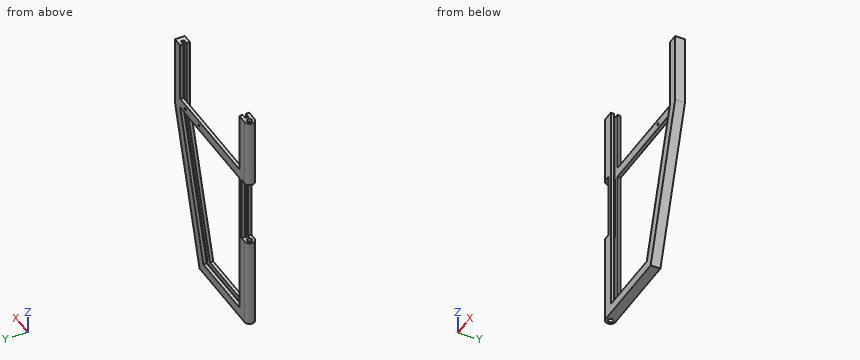
```python
from build123d import *

# Parameters (mm, degrees)
EXTRUDE_1_DEPTH                   = 3
SKETCH_2_R                        = 1.5
SKETCH_2_R_2                      = 0.75
EXTRUDE_2_DEPTH                   = 73
SKETCH_3_W                        = 42
SKETCH_3_H                        = 3.5
SKETCH_3_W_2                      = 3.2
SKETCH_3_H_2                      = 20.2
CUT_EXTRUDE_1_DEPTH               = 83.725086884
CUT_EXTRUDE_2_REACH               = 84.028
CUT_EXTRUDE_2_OFFSET_FROM_SURFACE = 1.5
CUT_EXTRUDE_START                 = -1.5
SKETCH_4_W                        = 44.5
SKETCH_4_H                        = 1
SKETCH_4_3_W                      = 22
SKETCH_4_3_H                      = 1
CUT_EXTRUDE_3_DEPTH               = 37.5
SKETCH_5_W                        = 3
SKETCH_5_H                        = 1
EXTRUDE_3_DEPTH                   = 34.5
SKETCH_6_R                        = 0.35
CUT_EXTRUDE_4_DEPTH               = 80.653562381
SKETCH_7_W                        = 24.036657481
SKETCH_7_H                        = 1
CUT_EXTRUDE_5_DEPTH               = 1.5


with BuildPart() as part:
    # 草图1 → 凸台-拉伸1 (new body)
    with BuildSketch(Plane(origin=(0, 0, 0), x_dir=(1, 0, 0), z_dir=(0, 1, 0))):
        Polygon((0, 0), (0, -73), (38.8, -73), (38.8, -47.5), (24.5, 0), align=None)
    extrude(amount=EXTRUDE_1_DEPTH)

    # 草图2 → 凸台-拉伸2 (add)
    # profile 1 of 2: a face of its own
    with BuildSketch(Plane(origin=(0, 0, 0), x_dir=(-1, 0, 0), z_dir=(0, 0, -1))):
        with BuildLine():
            Line((0, 3), (0, 0))
            Line((0, 0), (1.7, 0))
            ThreePointArc((1.7, 0), (0.2, 1.5), (1.7, 3))
            Line((1.7, 3), (0, 3))
        make_face()
    # profile 2 of 2: a face of its own
    with BuildSketch(Plane(origin=(0, 0, 0), x_dir=(-1, 0, 0), z_dir=(0, 0, -1))):
        with Locations((1.7, 1.5)):
            Circle(SKETCH_2_R)
        with Locations((1.7, 1.5)):
            Circle(SKETCH_2_R_2, mode=Mode.SUBTRACT)
    extrude(amount=-EXTRUDE_2_DEPTH)

    # 草图3 → 切除-拉伸1 (cut, through all)
    with BuildSketch(Plane(origin=(0, 3, 0), x_dir=(1, 0, 0), z_dir=(0, 1, 0))):
        with Locations((17.8, -71.25)):
            Rectangle(SKETCH_3_W, SKETCH_3_H)
        with Locations((-1.6, -38.1)):
            Rectangle(SKETCH_3_W_2, SKETCH_3_H_2)
        Polygon((1.3, -3), (22.270157068, -3), (35.8, -47.941785964), (35.8, -69.5), (1.3, -69.5), align=None)
    extrude(amount=-CUT_EXTRUDE_1_DEPTH, mode=Mode.SUBTRACT)

    # 切除-拉伸2: up to this face of the body (flat: up to its plane, moved by the offset)
    cut_extrude_2_end = Plane(part.part.faces().sort_by_distance((29.035078534, 1.5, 25.470892982))[0]).offset(-CUT_EXTRUDE_2_OFFSET_FROM_SURFACE)
    # 草图4 → 切除-拉伸2 (cut, up to the picked face)
    with BuildSketch(Plane(origin=(1.3, 0, 0), x_dir=(0, 0, -1), z_dir=(1, 0, 0)).offset(CUT_EXTRUDE_START), mode=Mode.PRIVATE) as cut_extrude_2_sk1:
        with Locations((-25.25, 1.5)):
            Rectangle(SKETCH_4_W, SKETCH_4_H)
    cut_extrude_2_tool1 = split(extrude(cut_extrude_2_sk1.sketch, amount=CUT_EXTRUDE_2_REACH, mode=Mode.PRIVATE), bisect_by=cut_extrude_2_end, keep=Keep.BOTH, mode=Mode.PRIVATE)
    add(cut_extrude_2_tool1.solids().sort_by(Axis((-0.2, 1.5, 25.25), (1, 0, 0)))[0], mode=Mode.SUBTRACT)

    # 草图4<3> → 切除-拉伸3 (cut)
    with BuildSketch(Plane(origin=(1.3, 0, 0), x_dir=(0, 0, -1), z_dir=(1, 0, 0)).offset(CUT_EXTRUDE_START)):
        with Locations((-58.5, 1.5)):
            Rectangle(SKETCH_4_3_W, SKETCH_4_3_H)
    extrude(amount=CUT_EXTRUDE_3_DEPTH, mode=Mode.SUBTRACT)

    # 草图5 → 凸台-拉伸3 (add)
    with BuildSketch(Plane.ZY.offset(-35.8)):
        with Locations((49.441785964, 2.5)):
            Rectangle(SKETCH_5_W, SKETCH_5_H)
    extrude(amount=EXTRUDE_3_DEPTH)

    # 草图6 → 切除-拉伸4 (cut, through all)
    with BuildSketch(Plane(origin=(0, 3, 0), x_dir=(1, 0, 0), z_dir=(0, 1, 0))):
        with Locations(Location((32.8, -49.441785964, 0), (0, 0, 270))):
            Circle(SKETCH_6_R)
        with Locations(Location((24.9, -49.441785964, 0), (0, 0, 270))):
            Circle(SKETCH_6_R)
    extrude(amount=-CUT_EXTRUDE_4_DEPTH, mode=Mode.SUBTRACT)

    # 草图7 → 切除-拉伸5 (cut)
    with BuildSketch(Plane.XY.offset(3)):
        with Locations((11.818328741, 1.5)):
            Rectangle(SKETCH_7_W, SKETCH_7_H)
    extrude(amount=-CUT_EXTRUDE_5_DEPTH, mode=Mode.SUBTRACT)


solid = part.part
```
Verification items for the finished model (mm, model axes). Coordinates: 2 decimals unless noted, no trailing zeros. Loops run counter-clockwise (first coordinate to the right, second up) from the corner with the lowest first, then second, coordinate; pieces in that order, holes last. Notation, with made-up numbers: (59, 23.5) - (98, 23.5) arc R15 ccw to (98, 52.5) - close; hole circle Ø1 at (52, -17.75). An arc over 180 degrees is marked (long way). Put each result on its own line as item: value.
Item 1: Scan lines: line 1 along Z through (x, y) = (4, 2.7); line 2 along Z through (x, y) = (21.5, 1.85); line 3 along X through (y, z) = (0.8, 40.5). Record each from-to range of solid material in increasing order.
Conclusion:
line 1: z = 0 to 3, 47.94 to 50.94
line 2: z = 0 to 1.5
line 3: x = 0 to 1.3, 33.56 to 36.69
Item 2: Section check A-A (z = 56). Enter the section's corners in (x, y), then the cut area to 3 significant figures.
Conclusion:
outline: (-1.7, 0) - (1.3, 0) - (1.3, 1) - (-0.2, 1) - (-0.2, 2) - (1.3, 2) - (1.3, 3) - (-1.7, 3) arc R1.5 ccw to start; (35.8, 0) - (38.8, 0) - (38.8, 3) - (35.8, 3) - (35.8, 2) - (37.3, 2) - (37.3, 1) - (35.8, 1) - close; hole circle Ø1.5 at (-1.7, 1.5)
area: 16.8 mm2
Item 3: Section check B-B (x = 18.5). Enter the section's corners in (y, z), then the cut area to 3 significant figures.
Conclusion:
outline: (0, 0) - (3, 0) - (3, 3) - (2, 3) - (2, 1.5) - (1, 1.5) - (1, 3) - (0, 3) - close; (2, 47.94) - (3, 47.94) - (3, 50.94) - (2, 50.94) - close
area: 10.5 mm2
Item 4: Section check D-D (z = 18.5). Enter the section's corners in (x, y), then the cut area to 3 significant figures.
Conclusion:
outline: (-1.7, 0) - (1.3, 0) - (1.3, 1) - (-0.2, 1) - (-0.2, 2) - (1.3, 2) - (1.3, 3) - (-1.7, 3) arc R1.5 ccw to start; (26.94, 0) - (30.07, 0) - (30.07, 3) - (26.94, 3) - (26.94, 2) - (28.5, 2) - (28.5, 1) - (26.94, 1) - close; hole circle Ø1.5 at (-1.7, 1.5)
area: 17.1 mm2
Item 5: Section check C-C (y = 1.5). Enter the section's corners in (x, z).
Conclusion:
outline: (-3.2, 0) - (-2.45, 0) - (-2.45, 28) - (-3.2, 28) - close; (-3.2, 48.2) - (-2.45, 48.2) - (-2.45, 69.5) - (-3.2, 69.5) - close; (-0.95, 0) - (24.5, 0) - (38.8, 47.5) - (38.8, 69.5) - (37.3, 69.5) - (37.3, 47.5) - (37.23, 47.5) - (23.84, 3) - (23.84, 1.5) - (-0.2, 1.5) - (-0.2, 28) - (-0.95, 28) - close; (-0.95, 48.2) - (-0.2, 48.2) - (-0.2, 69.5) - (-0.95, 69.5) - close
Item 6: Gauge pin test, flat ends, axial feed: pin 1 Ø11 at (x, z) = (23.5, 34) entering from -Y; pin 2 Ø0.5 at (y, z) = (2.5, 24.5) entering from +X; pin 3 Ø0.8 at (y, z) = (2.5, 40.5) entering from -X; pin 4 Ø8 at (x, z) = (22, 49) entering from -Y. Record the tip position at first contact, or that the pin passes through.
Conclusion:
pin 1: passes through
pin 2: stops at x = 31.95
pin 3: stops at x = 0
pin 4: stops at y = 2
